Could you check a few things on this model? Use its own coordinates, in mm. Face numbers are marked on the shaded views. A direction names the side the tool comes from. Coordinates: 2 decimals unless noted, no trailing zeros. Loops run counter-clockwise (first coordinate to the right, second up) from the corner with the lowest first, then second, coordinate; pieces in that order, holes last. Notation, with made-up numbers: (11.25, -27) -> (38.25, -27) arc R30 ccw to (38.25, -4) -> close; hole circle Ø11 at (-31.5, 33.25). An arc over 180 degrees is marked (long way). One line per question, with ' | ' between items.
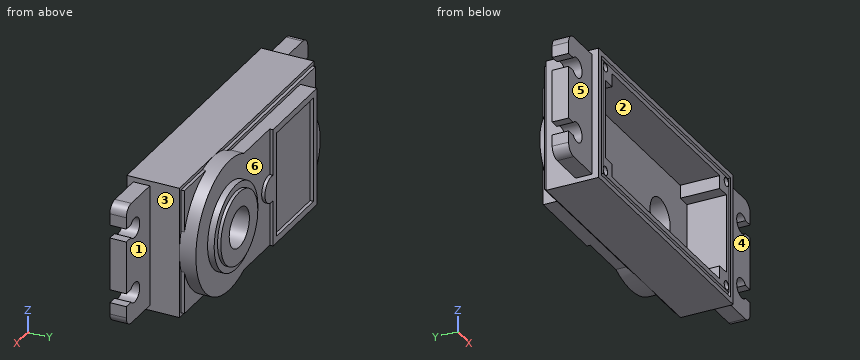
from build123d import *

# Parameters (mm, degrees)
SCHIZZO2_W                   = 40
SCHIZZO2_H                   = 20
ESTRUSIONE_ESTRUSIONE2_DEPTH = 8
TAGLIO_ESTRUSIONE4_DEPTH     = 6
ESTRUSIONE_ESTRUSIONE4_DEPTH = 2.5
SCHIZZO8_W                   = 39
SCHIZZO8_H                   = 19
ESTRUSIONE_ESTRUSIONE3_DEPTH = 0.5
SCHIZZO10_W                  = 11
SCHIZZO10_H                  = 16
ESTRUSIONE_ESTRUSIONE5_DEPTH = 0.5
SCHIZZO11_R                  = 6.5
ESTRUSIONE_ESTRUSIONE6_DEPTH = 1
SCHIZZO12_R                  = 5.5
ESTRUSIONE_ESTRUSIONE7_DEPTH = 0.5
SCHIZZO13_R                  = 3
TAGLIO_ESTRUSIONE5_DEPTH     = 26.377155081
SCHIZZO15_R                  = 1.5
ESTRUSIONE_ESTRUSIONE8_DEPTH = 2.5
SCHIZZO17_W                  = 7.322091749
SCHIZZO17_H                  = 2
TAGLIO_ESTRUSIONE6_DEPTH     = 31.020826105
SPECCHIA4_COPY_1_SKETCH_W    = 7.322091749
SPECCHIA4_COPY_1_SKETCH_H    = 2
SPECCHIA4_COPY_1_DEPTH       = 31.020826105


with BuildPart() as part:
    # Schizzo2 → Estrusione-Estrusione2 (new body)
    with BuildSketch(Plane(origin=(0, 0, 0), x_dir=(1, 0, 0), z_dir=(0, 1, 0))):
        Rectangle(SCHIZZO2_W, SCHIZZO2_H)
    extrude(amount=ESTRUSIONE_ESTRUSIONE2_DEPTH)

    # Schizzo3 → Taglio-Estrusione4 (cut)
    with BuildSketch(Plane(origin=(0, 0, 0), x_dir=(1, 0, 0), z_dir=(0, 1, 0))):
        Polygon((16, -8), (-16, -8), (-16, -6), (-18, -6), (-18, 6), (-16, 6), (-16, 8), (16, 8), (16, 6), (18, 6), (18, -6), (16, -6), align=None)
    extrude(amount=TAGLIO_ESTRUSIONE4_DEPTH, mode=Mode.SUBTRACT)

    # Schizzo4 → Foro per Vite M1-1 (revolve, cut)
    with BuildSketch(Plane(origin=(-18, 0, 8), x_dir=(0, 0, -1), z_dir=(1, 0, 0))):
        Polygon((0, 0), (0, 5.390559402), (0.65, 5), (0.65, 0.025), (0.675, 0), align=None)
    foro_per_vite_m1_1 = revolve(axis=Axis((-18, -6.35, 8), (0, 1, 0)), mode=Mode.SUBTRACT)

    # Specchia1: Foro per Vite M1-1 across plane
    add(foro_per_vite_m1_1.mirror(Plane(origin=(0, 0, 0), x_dir=(0, 0, 1), z_dir=(1, 0, 0))), mode=Mode.SUBTRACT)

    # Specchia2: Foro per Vite M1-1 across plane
    add(foro_per_vite_m1_1.mirror(Plane.XY), mode=Mode.SUBTRACT)

    # Specchia2 copy 1 sketch → Specchia2 copy 1 (revolve, cut)
    with BuildSketch(Plane(origin=(18, 0, -8), x_dir=(0, 0, 1), z_dir=(-1, 0, 0))):
        Polygon((0, 0), (0, 5.390559402), (0.65, 5), (0.65, 0.025), (0.675, 0), align=None)
    revolve(axis=Axis((18, -6.35, -8), (0, 1, 0)), mode=Mode.SUBTRACT)

    # Taglia-Sweep3: sweep along a path in Schizzo5
    with BuildLine(Plane.XZ) as taglia_sweep3_path:
        Line((19, -9), (-19, -9))
        Line((-19, -9), (-19, 9))
        Line((-19, 9), (19, 9))
        Line((19, 9), (19, -9))
    # Schizzo7 → Taglia-Sweep3 (sweep, cut)
    with BuildSketch(Plane.XY):
        with BuildLine():
            Line((-19.25, 0), (-18.75, 0))
            ThreePointArc((-18.75, 0), (-19, 0.25), (-19.25, 0))
        make_face()
    sweep(path=taglia_sweep3_path.line, transition=Transition.RIGHT, mode=Mode.SUBTRACT)

    # Schizzo9 → Estrusione-Estrusione4 (add)
    with BuildSketch(Plane(origin=(0, 8, 0), x_dir=(1, 0, 0), z_dir=(0, 1, 0))):
        with BuildLine():
            Line((5.641101056, 9), (-15, 9))
            Line((-15, 9), (-15, 5))
            ThreePointArc((-15, 5), (-17, 0), (-15, -5))
            Line((-15, -5), (-15, -9))
            Line((-15, -9), (5.641101056, -9))
            ThreePointArc((5.641101056, -9), (20, 0), (5.641101056, 9))
        make_face()
    extrude(amount=ESTRUSIONE_ESTRUSIONE4_DEPTH)

    # Schizzo8 → Estrusione-Estrusione3 (add)
    with BuildSketch(Plane(origin=(0, 8, 0), x_dir=(1, 0, 0), z_dir=(0, 1, 0))):
        Rectangle(SCHIZZO8_W, SCHIZZO8_H)
    extrude(amount=ESTRUSIONE_ESTRUSIONE3_DEPTH)

    # Schizzo10 → Estrusione-Estrusione5 (add)
    with BuildSketch(Plane(origin=(0, 10.5, 0), x_dir=(1, 0, 0), z_dir=(0, 1, 0))):
        with BuildLine():
            Line((-15, 9), (-2, 9))
            Line((-2, 9), (-2, 1.957707578))
            ThreePointArc((-2, 1.957707578), (0.409122281, 0), (-2, -1.957707578))
            Line((-2, -1.957707578), (-2, -9))
            Line((-2, -9), (-15, -9))
            Line((-15, -9), (-15, 9))
        make_face()
        with Locations((-8.5, 0)):
            Rectangle(SCHIZZO10_W, SCHIZZO10_H, mode=Mode.SUBTRACT)
    extrude(amount=ESTRUSIONE_ESTRUSIONE5_DEPTH)

    # Schizzo11 → Estrusione-Estrusione6 (add)
    with BuildSketch(Plane(origin=(0, 10.5, 0), x_dir=(1, 0, 0), z_dir=(0, 1, 0))):
        with Locations(Location((10, 0, 0), (0, 0, 270))):
            Circle(SCHIZZO11_R)
    extrude(amount=ESTRUSIONE_ESTRUSIONE6_DEPTH)

    # Schizzo12 → Estrusione-Estrusione7 (add)
    with BuildSketch(Plane(origin=(0, 11.5, 0), x_dir=(1, 0, 0), z_dir=(0, 1, 0))):
        with Locations(Location((10, 0, 0), (0, 0, 270))):
            Circle(SCHIZZO12_R)
    extrude(amount=ESTRUSIONE_ESTRUSIONE7_DEPTH)

    # Schizzo13 → Taglio-Estrusione5 (cut, through all)
    with BuildSketch(Plane(origin=(0, 12, 0), x_dir=(1, 0, 0), z_dir=(0, 1, 0))):
        with Locations(Location((10, 0, 0), (0, 0, 270))):
            Circle(SCHIZZO13_R)
    extrude(amount=-TAGLIO_ESTRUSIONE5_DEPTH, mode=Mode.SUBTRACT)

    # Schizzo15 → Estrusione-Estrusione8 (add)
    with BuildSketch(Plane(origin=(0, 1, 0), x_dir=(-1, 0, 0), z_dir=(0, -1, 0))):
        with BuildLine():
            Line((-25.5, 9.25), (-20, 9.25))
            Line((-20, 9.25), (-20, -9.25))
            Line((-20, -9.25), (-25.5, -9.25))
            ThreePointArc((-25.5, -9.25), (-26.560660172, -8.810660172), (-27, -7.75))
            Line((-27, -7.75), (-27, 7.75))
            ThreePointArc((-27, 7.75), (-26.560660172, 8.810660172), (-25.5, 9.25))
        make_face()
        with Locations(Location((-24.5, 5, 0), (0, 0, 90))):
            Circle(SCHIZZO15_R, mode=Mode.SUBTRACT)
        with Locations(Location((-24.5, -5, 0), (0, 0, 90))):
            Circle(SCHIZZO15_R, mode=Mode.SUBTRACT)
    estrusione_estrusione8 = extrude(amount=-ESTRUSIONE_ESTRUSIONE8_DEPTH)

    # Schizzo17 → Taglio-Estrusione6 (cut, through all)
    with BuildSketch(Plane(origin=(0, 3.5, 0), x_dir=(1, 0, 0), z_dir=(0, 1, 0))):
        with Locations((30.661045875, 5)):
            Rectangle(SCHIZZO17_W, SCHIZZO17_H)
        with BuildLine():
            Line((25.618033989, 4), (27, 4))
            Line((27, 4), (27, 6))
            Line((27, 6), (25.618033989, 6))
            ThreePointArc((25.618033989, 6), (25.645827846, 5.968028175), (25.672707741, 5.93528421))
            ThreePointArc((25.672707741, 5.93528421), (25.915814538, 5.495448478), (26, 5))
            ThreePointArc((26, 5), (25.915814538, 4.504551522), (25.672707741, 4.06471579))
            ThreePointArc((25.672707741, 4.06471579), (25.645827846, 4.031971825), (25.618033989, 4))
        make_face()
    taglio_estrusione6 = extrude(amount=-TAGLIO_ESTRUSIONE6_DEPTH, mode=Mode.SUBTRACT)

    # Specchia3: Taglio-Estrusione6 across plane
    add(taglio_estrusione6.mirror(Plane.XY), mode=Mode.SUBTRACT)

    # Specchia4: Estrusione-Estrusione8, Taglio-Estrusione6 across plane
    add(estrusione_estrusione8.mirror(Plane(origin=(0, 0, 0), x_dir=(0, 0, 1), z_dir=(1, 0, 0))))
    add(taglio_estrusione6.mirror(Plane(origin=(0, 0, 0), x_dir=(0, 0, 1), z_dir=(1, 0, 0))), mode=Mode.SUBTRACT)

    # Specchia4 copy 1 sketch → Specchia4 copy 1 (cut, through all)
    with BuildSketch(Plane(origin=(0, 3.5, 0), x_dir=(-1, 0, 0), z_dir=(0, 1, 0))):
        with Locations((30.661045875, 5)):
            Rectangle(SPECCHIA4_COPY_1_SKETCH_W, SPECCHIA4_COPY_1_SKETCH_H)
        with BuildLine():
            Line((25.618033989, 4), (27, 4))
            Line((27, 4), (27, 6))
            Line((27, 6), (25.618033989, 6))
            ThreePointArc((25.618033989, 6), (25.645827846, 5.968028175), (25.672707741, 5.93528421))
            ThreePointArc((25.672707741, 5.93528421), (25.915814538, 5.495448478), (26, 5))
            ThreePointArc((26, 5), (25.915814538, 4.504551522), (25.672707741, 4.06471579))
            ThreePointArc((25.672707741, 4.06471579), (25.645827846, 4.031971825), (25.618033989, 4))
        make_face()
    extrude(amount=-SPECCHIA4_COPY_1_DEPTH, mode=Mode.SUBTRACT)


solid = part.part
1) We'd pull the mould along X, two halves only. Please class the marked faces 1, 2 and 3: pulls with the +X half, pulls with the -X half, needs draft (parallel to the pull), parting line crosses it, or undercut.
Data:
face 1: needs draft | face 2: undercut | face 3: pulls with the +X half
2) On a 3-axis mill with a long thin cutter (end or side, diameter ignored), from which of +Z, -Z, +X, -X, +Y, -Y can I reach the whole of each face in a straight line? I mean the marked faces 4, 5 and 6. Say none if no direction works.
Data:
face 4: +Z, -Z, +X, -Y | face 5: +Z, -Z, -X, -Y | face 6: +Y
3) If we section it at A-A on y = 7: Please give me the cut outline in (x, z).
Data:
outline: (-20, -10) -> (20, -10) -> (20, 10) -> (-20, 10) -> close; hole circle Ø6 at (10, 0)
4) I need wall thicknesses on line 1 along Z through (x, y) = (16.5, 2.75); line 2 along Z through (x, y) = (-3.5, 3.25); line 3 along X through (y, z) = (5.25, 4). Which ranges of each line are inside material? Lowest first, please. Write a range as from..to.
Data:
line 1: -10..-6, 6..10 | line 2: -10..-8, 8..10 | line 3: -20..-18, 18..20
5) I'm going to push flat-ended pins straight in: pin 1 Ø3 at (y, z) = (8.5, 5.5) entering from +X; pin 2 Ø6 at (x, z) = (-21, 5) entering from +Y; pin 3 Ø1.5 at (x, y) = (26, 2) entering from +Z; pin 4 Ø5 at (x, z) = (-1.5, 6.5) entering from -Y. Where does each tip first touch, or does it pass through?
Data:
pin 1: x = 20 | pin 2: y = 8.5 | pin 3: z = 9.25 | pin 4: y = 0
6) If we section it at D-D on x = -20.5: Please give me the cut outline in (y, z), and give its area (4 significant figures).
Data:
outline: (1, -9.25) -> (3.5, -9.25) -> (3.5, 9.25) -> (1, 9.25) -> close | area: 46.25 mm²
7) If we section it at B-B on x = -9: Please give me the cut outline in (y, z).
Data:
outline: (0, -10) -> (8, -10) -> (8, -9.5) -> (8.5, -9.5) -> (8.5, -9) -> (11, -9) -> (11, -8) -> (10.5, -8) -> (10.5, 8) -> (11, 8) -> (11, 9) -> (8.5, 9) -> (8.5, 9.5) -> (8, 9.5) -> (8, 10) -> (0, 10) -> (0, 9.25) arc R0.25 cw to (0, 8.75) -> (0, 8) -> (6, 8) -> (6, -8) -> (0, -8) -> (0, -8.75) arc R0.25 cw to (0, -9.25) -> close
8) If we section it at C-C on y = 2.25: Give the number of separate pieces and of enclosed holes in the cut face, and give its area (3 significant figures).
Data:
separate pieces: 1 | enclosed holes: 5 | area: 455 mm²
